Read the model definition and answer for the solid it produces. Units are mm, in the model's axes. Give positions to 0.01 mm unless a question says otherwise; leave off trailing zeros. Loops run counter-clockwise (first coordinate to the right, second up) from the corner with the lowest first, then second, coordinate; pieces in that order, holes last. Notation, with made-up numbers: M 5,-19.5 L 55,-19.5 A37 ccw 55,17.5 Z; hole C -6,-32.5 d1. An arc over 180 degrees is marked long. Return JSON: item names as keys, results as strings. Group by question number.
```python
from build123d import *

# Parameters (mm, degrees)
SALIENTE_EXTRUIR1_DEPTH = 37
CORTAR_EXTRUIR1_DEPTH   = 11
CROQUIS4_W              = 5.3
CROQUIS4_H              = 39
CORTAR_EXTRUIR2_DEPTH   = 10
CORTAR_EXTRUIR3_DEPTH   = 7


with BuildPart() as part:
    # Croquis1 → Saliente-Extruir1 (new body)
    with BuildSketch(Plane.XY):
        Polygon((-99.889669891, -0.010626503), (-102.367816062, -1.441384861), (-103.432664129, -2.05617518), (-56.294122108, -83.702524956), (-52.829274, -81.702093968), (-52.153107423, -80.87251983), (-99.02316632, 0.48854437), align=None)
    extrude(amount=SALIENTE_EXTRUIR1_DEPTH)

    # Croquis2 → Cortar-Extruir1 (cut)
    with BuildSketch(Plane(origin=(-78.464848067, -45.301701153, 0), x_dir=(0, 0, 1), z_dir=(-0.866025404, -0.5, 0))):
        Polygon((4.142527364, -44.341451899), (4.142527364, -39.459427934), (0, -39.459427934), (-0.114610865, -39.459427934), (-0.114610865, -44.663143407), (4.142527364, -44.663143407), align=None)
        Polygon((34.863722121, -44.341451919), (34.863722121, -42.292638437), (37, -42.292638437), (37.495969664, -42.292638437), (37.495969664, -44.984834896), (34.863722121, -44.984834896), align=None)
    extrude(amount=-CORTAR_EXTRUIR1_DEPTH, mode=Mode.SUBTRACT)

    # Croquis4 → Cortar-Extruir2 (cut)
    with BuildSketch(Plane(origin=(-74.09577594, -42.782555705, 0), x_dir=(0, 0, 1), z_dir=(-0.866503572, -0.499170873, 0))):
        with Locations((30.774409531, 0.000869875)):
            Rectangle(CROQUIS4_W, CROQUIS4_H)
    extrude(amount=CORTAR_EXTRUIR2_DEPTH, mode=Mode.SUBTRACT)

    # Croquis5 → Cortar-Extruir3 (cut)
    with BuildSketch(Plane(origin=(-74.09577594, -42.782555705, 0), x_dir=(0, 0, 1), z_dir=(-0.866503572, -0.499170873, 0))):
        Polygon((28.224409531, 7.991554704), (26.034587607, 7.991554704), (26.034587607, 5.602236085), (23.516116629, 5.602236085), (23.516116629, -3.658890685), (26.034587607, -3.658890685), (26.034587607, -6.048209304), (28.224409531, -6.048209304), (28.726361193, -6.048209304), (28.726361193, 7.991554704), align=None)
    extrude(amount=CORTAR_EXTRUIR3_DEPTH, mode=Mode.SUBTRACT)


solid = part.part
```
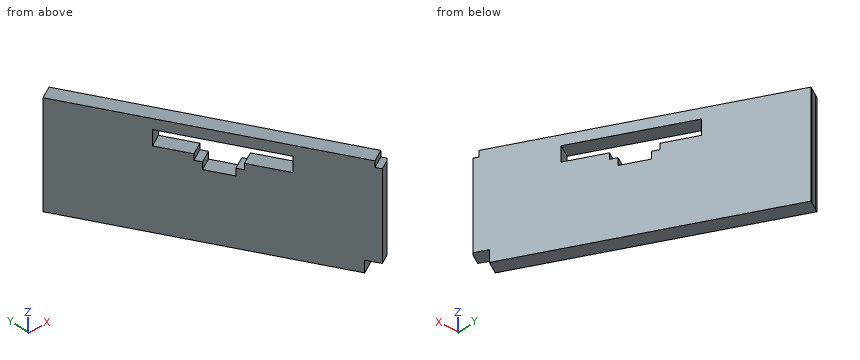
1. Straight lines are drawn through the part: line 1 along Z through (x, y) = (-70, -58.5); line 2 along Y through (x, z) = (-69.5, 10.5); line 3 along Y through (x, z) = (-72.5, 21). For each, find the intervals that lie inside material, in ascending order.
2. Flat-ended cylindrical pins translate along their axes: P1, Ø3, axis at x = -78.5, z = 28, coming from the -Y side; P2, Ø1.5, axis at x = -87.5, z = 28, coming from the -Y side; P3, Ø8, axis at x = -64.5, z = 15, coming from the -Y side. Find the tip coordinate at first contact, or state that the pin passes through.
3. Find section D-D (y = -22). Write down the section's boundary in (x, z).
4. Find section A-A (z = 29.5). Write down the section's boundary in (x, y), and give its area (3 significant figures).
5. Find section B-B (y = -57). Write down the section's boundary in (x, z), and give its area (3 significant figures).
6. Find section C-C (z = 20.5). Write down the section's boundary in (x, y).
Result:
{
 "1": {"line 1": "z = 0 to 28.12, 33.42 to 37", "line 2": "y = -60.83 to -50.76", "line 3": "y = -55.63 to -45.55"},
 "2": {"P1": "stops at y = -36.96", "P2": "stops at y = -30.95", "P3": "stops at y = -76.42"},
 "3": {"outline": "M -91.92,0 L -86.07,0 L -86.07,37 L -91.92,37 Z"},
 "4": {"outline": "M -103.43,-2.06 L -88.22,-28.41 L -83.83,-25.88 L -99.02,0.49 L -99.89,-0.01 Z; M -68.72,-62.19 L -56.29,-83.7 L -52.83,-81.7 L -52.15,-80.87 L -64.36,-59.68 Z", "area": "279 mm2"},
 "5": {"outline": "M -71.71,0 L -65.91,0 L -65.91,28.12 L -71.71,28.12 Z; M -71.71,33.42 L -65.91,33.42 L -65.91,37 L -71.71,37 Z", "area": "184 mm2"},
 "6": {"outline": "M -103.43,-2.06 L -56.29,-83.7 L -52.83,-81.7 L -52.15,-80.87 L -99.02,0.49 L -99.89,-0.01 Z"}
}
